Can you work these out from the model? Positions are in its coordinate system, mm. A direction names the side the tool comes from. Give positions to 0.01 mm unless a question says otherwise; leave off trailing zeros. Order: outer loops, then holes, each group sorted by start corner. A loop starts at its lowest first (then second) coordinate and runs counter-clockwise, first axis right, second up. Notation, with made-up numbers: (79, 4) -> (89, 4) arc R15 cw to (89, 15) -> close; hole circle Ø9 at (39, 53.25). An arc over 180 degrees is marked (long way). Answer as a JSON object with one key per item and string values.
```python
from build123d import *

# Parameters (mm, degrees)
SKETCH1_W           = 10
SKETCH1_H           = 108
BOSS_EXTRUDE1_DEPTH = 5
SKETCH2_R           = 1.75
CUT_EXTRUDE1_DEPTH  = 109.231233939
BOSS_EXTRUDE2_DEPTH = 5
SKETCH5_R           = 2.2
CUT_EXTRUDE2_DEPTH  = 5
BOSS_EXTRUDE3_REACH = 128.484
BOSS_EXTRUDE4_DEPTH = 8
SKETCH8_R           = 1.75
CUT_EXTRUDE3_DEPTH  = 129.116541509


with BuildPart() as part:
    # Sketch1 → Boss-Extrude1 (new body)
    with BuildSketch(Plane.XY):
        with Locations((0, 54)):
            Rectangle(SKETCH1_W, SKETCH1_H)
    extrude(amount=BOSS_EXTRUDE1_DEPTH)

    # Sketch2 → Cut-Extrude1 (cut, through all)
    with BuildSketch(Plane.XY.offset(5)):
        with Locations((0, 10)):
            Circle(SKETCH2_R)
        with Locations((0, 103)):
            Circle(SKETCH2_R)
    extrude(amount=-CUT_EXTRUDE1_DEPTH, mode=Mode.SUBTRACT)

    # Sketch4 → Boss-Extrude2 (add)
    with BuildSketch(Plane(origin=(0, 49.1, 0), x_dir=(-1, 0, 0), z_dir=(0, -1, 0))):
        Polygon((3.377813163, 0), (40.9972684, 27.282007374), (40.703728886, 27.686772187), (51.227614019, 35.318799552), (55.63070673, 29.247327359), (45.106791947, 21.615278492), (43.932633891, 23.234337744), (5, -5), align=None)
    extrude(amount=-BOSS_EXTRUDE2_DEPTH)

    # Sketch5 → Cut-Extrude2 (cut)
    with BuildSketch(Plane.XZ.offset(-49.1)):
        with Locations((-47.97, -29.25)):
            Circle(SKETCH5_R)
    extrude(amount=-CUT_EXTRUDE2_DEPTH, mode=Mode.SUBTRACT)

    # Boss-Extrude3: up to this face of the body (flat: up to its plane)
    boss_extrude3_end = Plane(part.part.faces().sort_by_distance((-22.187540781, 51.6, -13.641003687))[0])
    # Sketch6 → Boss-Extrude3 (add, up to the picked face)
    with BuildSketch(Plane(origin=(-4.099598255, 0, 5.652980403), x_dir=(0.8095296256563876, 0, 0.5870790280572362), z_dir=(-0.5870790280572362, 0, 0.8095296256563876)), mode=Mode.PRIVATE) as boss_extrude3_sk1:
        Polygon((-43.1833208, 54.1), (-1.112252988, 96.171067812), (-1.112252988, 89.1), (-36.112252988, 54.1), align=None)
    boss_extrude3_tool1 = split(extrude(boss_extrude3_sk1.sketch, amount=-BOSS_EXTRUDE3_REACH, mode=Mode.PRIVATE), bisect_by=boss_extrude3_end, keep=Keep.BOTH, mode=Mode.PRIVATE)
    add(boss_extrude3_tool1.solids().sort_by(Axis((-20.641593, 73.42183, -6.343441), (0.5870790280572362, 0, -0.8095296256563876)))[0])

    # Sketch7 → Boss-Extrude4 (add)
    with BuildSketch(Plane(origin=(0, 54.1, 0), x_dir=(1, 0, 0), z_dir=(0, 1, 0))):
        Polygon((-40.645020983, 27.767725149), (-52.102962866, 39.221816124), (-58.059295607, 31.008564443), (-45.106791947, 21.615278492), align=None)
    extrude(amount=BOSS_EXTRUDE4_DEPTH)

    # Sketch8 → Cut-Extrude3 (cut, through all)
    with BuildSketch(Plane(origin=(-6.431817345, 0, 6.433979746), x_dir=(-0.7072256172064263, 0, -0.7069879251917881), z_dir=(0.7069879251917881, 0, -0.7072256172064263))):
        with Locations((58.876646442, 58.1)):
            Circle(SKETCH8_R)
    extrude(amount=-CUT_EXTRUDE3_DEPTH, mode=Mode.SUBTRACT)


solid = part.part
```
1. If we mould it in two halves opening along Z, with no side actions, what happens to faces 1 (the face through (-52.098, 59.576, -32.493)), 2 (the face through (-20.82, 74.84, -9.52)), 3 (the face through (-0.38, 101.29, 2.54)), 4 (the face through (-46.95, 51.56, -31.2))? For each: +Z half, -Z half, draft (parallel to the pull), parting line (faces both ways), or undercut.
Worked answers:
{"face 1": "undercut", "face 2": "-Z half", "face 3": "draft", "face 4": "undercut"}
2. Will these pins go through, and if not, where does the flat tip stop? pin 1 Ø5 at (y, z) = (65, -0.5) entering from +X; pin 2 Ø2.5 at (x, z) = (-42, -25) entering from +Y; pin 3 Ø5.5 at (y, z) = (19.5, 2) entering from -X; pin 4 Ø19.5 at (x, z) = (-14.5, -13) entering from +Y.
Worked answers:
{"pin 1": "x = 5", "pin 2": "y = 62.1", "pin 3": "x = -5", "pin 4": "y = 86.81"}
3. If we section it at B-B on x = 0: Please give me the cut outline in (y, z).
Worked answers:
{"outline": "(0, 0) -> (8.25, 0) -> (8.25, 5) -> (0, 5) -> close; (11.75, 0) -> (101.25, 0) -> (101.25, 5) -> (11.75, 5) -> close; (104.75, 0) -> (108, 0) -> (108, 5) -> (104.75, 5) -> close"}
4. For faces 5 (the face through (-5, 101, 2)), 6 (the face through (-40, 54.1, -24)), 7 (the face through (-49, 62.1, -31)), 8 (the face through (-53.398, 51.565, -32.326)), which set-ups out of +Z, -Z, +X, -X, +Y, -Y let a thin tool reach every point of the face, with its end or its side?
Worked answers:
{"face 5": "-Z, -X, +Y", "face 6": "+Y", "face 7": "+Z, -Z, +X, -X, +Y", "face 8": "-Z, -X, -Y"}
5. Please list where these lines run through material, in increasing order: L1, parallel to Y at x = 0, z = 2; L2, parallel to X at y = 103, z = 1.5; L3, parallel to Z at x = -47.97, y = 50.4.
Worked answers:
{"L1": "0 to 8.25, 11.75 to 101.25, 104.75 to 108", "L2": "-5 to -1.75, 1.75 to 5", "L3": "-32.96 to -31.45, -27.05 to -23.69"}
6. If we section it at A-A on y = 103: Please give me the cut outline in (x, z), then the cut area to 3 significant figures.
Worked answers:
{"outline": "(-5, 0) -> (-1.75, 0) -> (-1.75, 5) -> (-5, 5) -> close; (1.75, 0) -> (5, 0) -> (5, 5) -> (1.75, 5) -> close", "area": "32.5 mm²"}
7. If we section it at D-D on y = 19.5: Please give me the cut outline in (x, z).
Worked answers:
{"outline": "(-5, 0) -> (5, 0) -> (5, 5) -> (-5, 5) -> close"}
8. If we section it at C-C on z = -13: Please give me the cut outline in (x, y), then the cut area to 3 significant figures.
Worked answers:
{"outline": "(-29.82, 49.1) -> (-21.3, 49.1) -> (-21.3, 54.1) -> (-29.82, 54.1) -> close; (-29.82, 58.44) -> (-21.3, 65.33) -> (-21.3, 72.41) -> (-29.82, 65.51) -> close", "area": "103 mm²"}
